from build123d import *

# Parameters (mm, degrees)
BOSS_EXTRUDE1_DEPTH     = 10
CUT_EXTRUDE1_DEPTH      = 21.976176963
CUT_EXTRUDE1_DEPTH_BACK = 10
SKETCH2_OUTSIDE_W       = 45.568
SKETCH2_OUTSIDE_H       = 19.568
M2_CLEARANCE_HOLE1_D    = 2.4


with BuildPart() as part:
    # Sketch1 → Boss-Extrude1 (new body)
    with BuildSketch(Plane(origin=(0, 0, 0), x_dir=(1, 0, 0), z_dir=(0, 1, 0))):
        with BuildLine():
            Line((2, -12.171572875), (2, 12.171572875))
            ThreePointArc((2, 12.171572875), (1, 18), (0, 12.171572875))
            Line((0, 12.171572875), (0, -12.171572875))
            ThreePointArc((0, -12.171572875), (1, -18), (2, -12.171572875))
        make_face()
    extrude(amount=BOSS_EXTRUDE1_DEPTH)

    # Sketch2 outside → Cut-Extrude1 (cut, two sides: drawn at the far end of the back side and taken through both)
    with BuildSketch(Plane(origin=(2, 0, 0), x_dir=(0, 0, -1), z_dir=(1, 0, 0)).offset(-CUT_EXTRUDE1_DEPTH_BACK)):
        with Locations((0, 5)):
            Rectangle(SKETCH2_OUTSIDE_W, SKETCH2_OUTSIDE_H)
        Polygon((6.57130649, 4), (-6.57130649, 4), (-12.171572875, 1), (-12.171572875, 0), (-18, 0), (-18, 2), (-12.422546375, 2), (-6.822279989, 5), (6.822279989, 5), (12.422546375, 2), (18, 2), (18, 0), (12.171572875, 0), (12.171572875, 1), align=None, mode=Mode.SUBTRACT)
    extrude(amount=CUT_EXTRUDE1_DEPTH + CUT_EXTRUDE1_DEPTH_BACK, mode=Mode.SUBTRACT)

    # M2 Clearance Hole1 (through all)
    with Locations(Plane(origin=(0, 2, 0), x_dir=(1, 0, 0), z_dir=(0, 1, 0))):
        with Locations((1, 15), (1, -15)):
            Hole(M2_CLEARANCE_HOLE1_D / 2)


solid = part.part
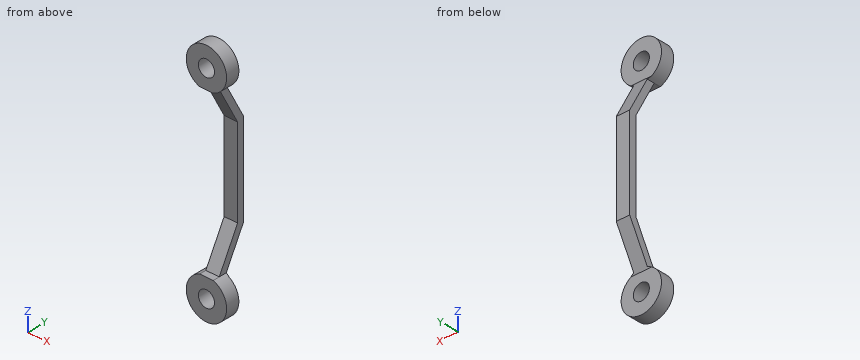
Geometry check sheet. Reference: the model listing, model coordinates, mm. Coordinates: 2 decimals unless noted, no trailing zeros. Order: outer loops, then holes, each group sorted by start corner. A loop starts at its lowest first (then second) coordinate and runs counter-clockwise, first axis right, second up. Notation, with made-up numbers: (-34.75, -17.75) - (15.25, -17.75) arc R14 ccw to (15.25, -6.75) - close; hole circle Ø7 at (-37, 75.25). An arc over 180 degrees is marked (long way). Answer in a Markdown table with one row per item. Add a question column.
1) Cross-section at B-B, the plane x = 1. Record the cut outline in (y, z).
2) Gauge pin test, flat ends, axial feed: P1, Ø2, axis at x = 0.5, z = 2.5, coming from the -Y side; P2, Ø3, axis at y = 3.5, z = -5, coming from the -X side; P3, Ø3, axis at x = 1, z = -15, coming from the -Y side; P4, Ø3, axis at x = 2.5, z = 9.5, coming from the -Y side. Record the tip position at first contact, or that the pin passes through.
3) Cross-section at A-A, the plane z = -15. Record the cut outline in (x, y), then the cut area to 3 significant figures.
4) Cross-section at C-C, the plane y = 1.55. Record the cut outline in (x, z), then the cut area to 3 significant figures.
5) Material ranges on line 1 along X through (y, z) = (1.1, 15); line 2 along Z through (x, y) = (1, 0.55); line 3 along Z through (x, y) = (1, 1.05), recorded low to high. Write a range as [from, to].
6) Cross-section at D-D, the plane x = -1.5. Record the cut outline in (y, z), then the cut area to 3 significant figures.
Check result:
| question | item | result |
|---|---|---|
| 1 | outline | (0, -18) - (2, -18) - (2, -16.2) - (0, -16.2) - close; (0, -13.8) - (2, -13.8) - (2, -12.42) - (5, -6.82) - (5, 6.82) - (2, 12.42) - (2, 13.8) - (0, 13.8) - (0, 12.17) - (1, 12.17) - (4, 6.57) - (4, -6.57) - (1, -12.17) - (0, -12.17) - close; (0, 16.2) - (2, 16.2) - (2, 18) - (0, 18) - close |
| 2 | P1 | stops at y = 4 |
| 2 | P2 | stops at x = 0 |
| 2 | P3 | stops at y = 0 |
| 2 | P4 | stops at y = 1.67 |
| 3 | outline | (-2, 0) - (-0.2, 0) - (-0.2, 2) - (-2, 2) - close; (2.2, 0) - (4, 0) - (4, 2) - (2.2, 2) - close |
| 3 | area | 7.20 mm² |
| 4 | outline | (0, -12.17) arc R3 ccw (long way) to (2, -12.17) - (2, -11.14) - (0, -11.14) - close; (0, 11.14) - (2, 11.14) - (2, 12.17) arc R3 ccw (long way) to (0, 12.17) - close; hole circle Ø2.4 at (1, -15); hole circle Ø2.4 at (1, 15) |
| 4 | area | 51.1 mm² |
| 5 | line 1 | x = [-2, -0.2], [2.2, 4] |
| 5 | line 2 | z = [-18, -16.2], [-13.8, -12.17], [12.17, 13.8], [16.2, 18] |
| 5 | line 3 | z = [-18, -16.2], [-13.8, -12.08], [12.08, 13.8], [16.2, 18] |
| 6 | outline | (0, -16.66) - (2, -16.66) - (2, -13.34) - (0, -13.34) - close; (0, 13.34) - (2, 13.34) - (2, 16.66) - (0, 16.66) - close |
| 6 | area | 13.3 mm² |
